Input: part model. Units: mm. Frame: model coordinates. Face numbers are marked on the shaded views. A direction names the side the tool comes from. Coordinates: 2 decimals unless noted, no trailing zeros. Loops run counter-clockwise (first coordinate to the right, second up) from the corner with the lowest first, then second, coordinate; pieces in that order, holes last. Notation, with made-up numbers: M -8.75,-7 L 11.25,-7 A24 ccw 11.25,26 Z; hole C 63.5,7 d5. An arc over 180 degrees is marked long. Use a Markdown table: item, result. Add a question column.
1. Section A-A on y = -42.5. Output: boundary loops of the cut face in (x, z), then the cut area to 3 significant figures.
2. Section B-B on x = 22. Output: boundary loops of the cut face in (y, z).
3. Draft query along X for the marked faces 6, 7 and 8. Return one class per face: +X half, -X half, draft (parallel to the pull), parting line (faces both ways), or undercut.
4. Set-up query: the marked faces 1, 2, 3, 4 and 5. Return all of +Z, -Z, +X, -X, +Y, -Y with unobstructed straight access to the full face (end or side cutting, diameter ignored); none if empty.
5. Pin query (flat end, axial travel): pin 1 (3 mm diameter, centred on y = -36, z = 2, fed in from -X); pin 2 (21 mm diameter, centred on x = 77, z = 28, fed in from -Y); pin 3 (10 mm diameter, centred on x = 91, z = 39.5, fed in from +Y). Return the tip coordinate at first contact, or that it passes through.
6. Line query: L1, parallel to Z at x = 22, y = -44; L2, parallel to Y at x = 29, z = 52.5; L3, parallel to Z at x = 63, y = -34. Output: solid intervals per line, ascending. Write a range as [from, to].
7. Section D-D on y = -8. Output: boundary loops of the cut face in (x, z), then the cut area to 3 significant figures.
8. Section C-C on z = 28. Output: boundary loops of the cut face in (x, y).
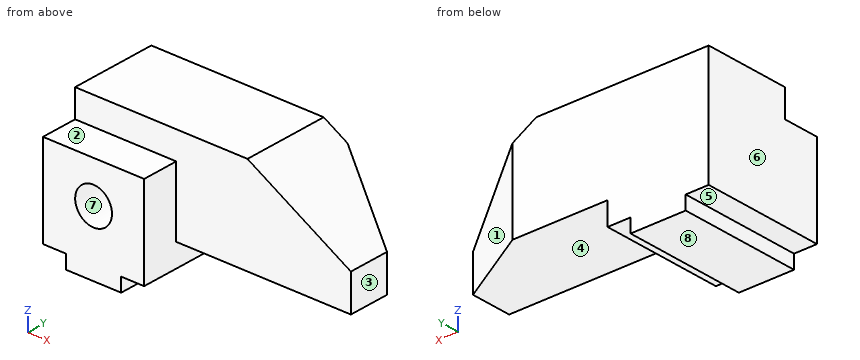
```python
from build123d import *

# Parameters (mm, degrees)
F0_W     = 44
F0_H     = 30
F0_R     = 8
F1_DEPTH = 54
F2_DEPTH = 38
F3_R     = 8
F4_DEPTH = 22
F6_DEPTH = 42.001


with BuildPart() as f1:
    # F0 (on Front) → F1 (new body)
    with BuildSketch(Plane.XZ):
        Polygon((0, 16), (0, 6), (10, 6), (10, 0), (34, 0), (34, 6), (44, 6), (44, 16), align=None)
        with Locations((22, 31)):
            Rectangle(F0_W, F0_H)
        with Locations((22, 28)):
            Circle(F0_R, mode=Mode.SUBTRACT)
        with Locations((22, 28)):
            Circle(F0_R)
    extrude(amount=F1_DEPTH)

    # F0 (on Front) → F2 (join)
    with BuildSketch(Plane.XZ):
        Polygon((0, 58), (0, 46), (44, 46), (44, 16), (120, 16), (120, 32.019238), (75, 58), align=None)
    extrude(amount=F2_DEPTH)

    # F3 (on face) → F4 (cut)
    with BuildSketch(Plane.XZ.offset(54)):
        with Locations((22, 28)):
            Circle(F3_R)
    extrude(amount=-F4_DEPTH, mode=Mode.SUBTRACT)

    # F5 (on face) → F6 (cut, through all)
    with BuildSketch(Plane(origin=(0, 0, 16), x_dir=(1, 0, 0), z_dir=(0, 0, -1))):
        Polygon((85.358984, 0), (120, 0), (120, 20), align=None)
    extrude(amount=-F6_DEPTH, mode=Mode.SUBTRACT)


solid = f1.part
```
Answers below:
| question | item | result |
|---|---|---|
| 1 | outline | M 0,6 L 10,6 L 10,0 L 34,0 L 34,6 L 44,6 L 44,46 L 0,46 Z; hole C 22,28 d16 |
| 1 | area | 1,700 mm² |
| 2 | outline | M -54,0 L 0,0 L 0,58 L -38,58 L -38,46 L -54,46 L -54,36 L -32,36 L -32,20 L -54,20 Z |
| 3 | face 6 | -X half |
| 3 | face 7 | undercut |
| 3 | face 8 | draft |
| 4 | face 1 | +Z, -Z, +X, +Y |
| 4 | face 2 | +Z, +X, -X, -Y |
| 4 | face 3 | +Z, -Z, +X, +Y, -Y |
| 4 | face 4 | -Z, +X, +Y, -Y |
| 4 | face 5 | -Z, -X, +Y, -Y |
| 5 | pin 1 | stops at x = 10 |
| 5 | pin 2 | stops at y = -38 |
| 5 | pin 3 | stops at y = -0.37 |
| 6 | L1 | z = [0, 20], [36, 46] |
| 6 | L2 | y = [-38, 0] |
| 6 | L3 | z = [16, 58] |
| 7 | outline | M 0,6 L 10,6 L 10,0 L 34,0 L 34,6 L 44,6 L 44,16 L 99.22,16 L 99.22,44.02 L 75,58 L 0,58 Z |
| 7 | area | 4,580 mm² |
| 8 | outline | M 0,-54 L 14,-54 L 14,-32 L 30,-32 L 30,-54 L 44,-54 L 44,-38 L 120,-38 L 120,-20 L 85.36,0 L 0,0 Z |
